from build123d import *

# Parameters (mm, degrees)
BOSS_EXTRUDE1_DEPTH = 6
SKETCH2_R           = 1.75
CUT_EXTRUDE1_DEPTH  = 6.6
FILLET1_R           = 0.5
SKETCH3_W           = 3.4
SKETCH3_H           = 5
BOSS_EXTRUDE2_DEPTH = 5
FILLET2_R           = 1
SKETCH5_R           = 1.75
CUT_EXTRUDE2_DEPTH  = 4
FILLET3_R           = 1


with BuildPart() as part:
    # Sketch1 → Boss-Extrude1 (new body)
    with BuildSketch(Plane.XY):
        with BuildLine():
            Line((0.5, 0), (6.1, 0))
            ThreePointArc((6.1, 0), (6.453553391, 0.146446609), (6.6, 0.5))
            Line((6.6, 0.5), (6.6, 4.5))
            ThreePointArc((6.6, 4.5), (6.453553391, 4.853553391), (6.1, 5))
            Line((6.1, 5), (0.5, 5))
            ThreePointArc((0.5, 5), (0.146446609, 4.853553391), (0, 4.5))
            Line((0, 4.5), (0, 0.5))
            ThreePointArc((0, 0.5), (0.146446609, 0.146446609), (0.5, 0))
        make_face()
    extrude(amount=BOSS_EXTRUDE1_DEPTH)

    # Sketch2 → Cut-Extrude1 (cut)
    with BuildSketch(Plane(origin=(6.6, 0, 0), x_dir=(0, 0, -1), z_dir=(1, 0, 0))):
        with Locations((-2.75, 2.5)):
            Circle(SKETCH2_R)
    extrude(amount=-CUT_EXTRUDE1_DEPTH, mode=Mode.SUBTRACT)

    # Fillet1
    fillet1_edges = [part.edges().sort_by_distance(p)[0] for p in [
        (0, 2.5, 0),
        (0.146446609, 4.853553391, 0),
        (3.3, 5, 0),
        (6.453553391, 4.853553391, 0),
        (6.6, 2.5, 0),
        (6.453553391, 0.146446609, 0),
        (3.3, 0, 0),
        (0.146446609, 0.146446609, 0),
    ]]
    fillet(fillet1_edges, radius=FILLET1_R)

    # Sketch3 → Boss-Extrude2 (add)
    with BuildSketch(Plane.XY.offset(6)):
        with Locations((3.3, 2.5)):
            Rectangle(SKETCH3_W, SKETCH3_H)
    extrude(amount=BOSS_EXTRUDE2_DEPTH)

    # Fillet2
    fillet2_edges = [part.edges().sort_by_distance(p)[0] for p in [
        (1.6, 2.5, 6),
        (5, 2.5, 6),
    ]]
    fillet(fillet2_edges, radius=FILLET2_R)

    # Sketch5 → Cut-Extrude2 (cut)
    with BuildSketch(Plane(origin=(5, 0, 0), x_dir=(0, 0, -1), z_dir=(1, 0, 0))):
        with Locations(Location((-9, 2.5, 0), (0, 0, 90))):
            Circle(SKETCH5_R)
    extrude(amount=-CUT_EXTRUDE2_DEPTH, mode=Mode.SUBTRACT)

    # Fillet3
    fillet3_edges = [part.edges().sort_by_distance(p)[0] for p in [
        (3.3, 5, 11),
        (3.3, 0, 11),
    ]]
    fillet(fillet3_edges, radius=FILLET3_R)


solid = part.part
Could you check a few things on this model? Use its own coordinates, in mm. A direction names the side the tool comes from. Coordinates: 2 decimals unless noted, no trailing zeros. Order: outer loops, then holes, each group sorted by start corner. A loop starts at its lowest first (then second) coordinate and runs counter-clockwise, first axis right, second up. Notation, with made-up numbers: (9.5, 75) - (21.5, 75) arc R11 ccw to (21.5, 83) - close; hole circle Ø5 at (-8.5, -27.5). An arc over 180 degrees is marked (long way). Answer in a Markdown table with one row per item. Add a question column.
(1) On a 3-axis mill with a long thin cutter (end or side, diameter ignored), from which of +Z, -Z, +X, -X, +Y, -Y can I reach the whole of each face in a straight line? I mean faces 1 (the face through (1.6, 1.91, 7.19)), 2 (the face through (5, 1.91, 7.19)), 3 (the face through (6.6, 1.58, 4.43)). Say none if no direction works.
(2) If we section it at B-B, the plane z = 9: Please give me the cut outline in (x, y).
(3) If we section it at C-C, the plane x = 2: Please give me the cut outline in (y, z).
(4) If we section it at A-A, the plane y = 2.5: Please give me the cut outline in (x, z).
(5) If we section it at D-D, the plane x = 1.25: Please give me the cut outline in (y, z).
(6) I need wall thicknesses on L1, parallel to Y at x = 4.5, z = 2.75; L2, parallel to Z at x = 4.5, y = 2; L3, parallel to Z at x = 2.5, y = 1.8. Which ranges of each line are inside material? Lowest first, please.
(7) If we mould it in two halves opening along Y, with no side actions, what happens to faces 4 (the face through (3.324, 0.285, 10.699)), 5 (the face through (3, 3, 0)), 6 (the face through (3.324, 4.699, 10.715)), 7 (the face through (3.35, 0.95, 1.94))? For each: released by +Y, released by -Y, zero draft, split by the parting line, or undercut.
(8) Will these pins go through, and if not, where does the flat tip stop? pin 1 (2 mm diameter, centred on y = 3, z = 8.5, fed in from +X); pin 2 (0.5 mm diameter, centred on x = 6, y = 3, fed in from +Z); pin 3 (2 mm diameter, centred on x = 5.5, y = 4, fed in from +Z).
Results are:
| question | item | result |
|---|---|---|
| 1 | face 1 | +Z, -X, +Y, -Y |
| 1 | face 2 | +Z, +X, +Y, -Y |
| 1 | face 3 | +Z, -Z, +X, +Y, -Y |
| 2 | outline | (1.6, 0) - (5, 0) - (5, 0.75) - (1.6, 0.75) - close; (1.6, 4.25) - (5, 4.25) - (5, 5) - (1.6, 5) - close |
| 3 | outline | (0, 0.5) arc R0.5 ccw to (0.5, 0) - (4.5, 0) arc R0.5 ccw to (5, 0.5) - (5, 10) arc R1 ccw to (4, 11) - (1, 11) arc R1 ccw to (0, 10) - close; hole circle Ø3.5 at (2.5, 2.75); hole circle Ø3.5 at (2.5, 9) |
| 4 | outline | (0, 0.5) arc R0.5 ccw to (0.5, 0) - (6.1, 0) arc R0.5 ccw to (6.6, 0.5) - (6.6, 1) - (0, 1) - close; (0, 4.5) - (6.6, 4.5) - (6.6, 6) - (6, 6) arc R1 cw to (5, 7) - (5, 7.25) - (1.6, 7.25) - (1.6, 7) arc R1 cw to (0.6, 6) - (0, 6) - close; (1.6, 10.75) - (5, 10.75) - (5, 11) - (1.6, 11) - close |
| 5 | outline | (0, 0.5) arc R0.5 ccw to (0.5, 0) - (4.5, 0) arc R0.5 ccw to (5, 0.5) - (5, 6.24) - (0, 6.24) - close; hole circle Ø3.5 at (2.5, 2.75) |
| 6 | L1 | y = 0 to 0.75, 4.25 to 5 |
| 6 | L2 | z = 0 to 1.07, 4.43 to 7.32, 10.68 to 11 |
| 6 | L3 | z = 0 to 1.15, 4.35 to 7.4, 10.6 to 11 |
| 7 | face 4 | released by -Y |
| 7 | face 5 | zero draft |
| 7 | face 6 | released by +Y |
| 7 | face 7 | undercut |
| 8 | pin 1 | passes through |
| 8 | pin 2 | stops at z = 6.03 |
| 8 | pin 3 | stops at z = 11 |
